```python
from build123d import *

# Parameters (mm, degrees)
SKETCH1_W                = 25.5
SKETCH1_H                = 42
BOSS_EXTRUDE1_DEPTH      = 5.5
SKETCH2_W                = 25
SKETCH2_H                = 36
CUT_EXTRUDE1_DEPTH       = 3
SKETCH3_R                = 10.5
CUT_EXTRUDE6_DEPTH       = 29
SKETCH6_R                = 2.75
CUT_EXTRUDE7_DEPTH       = 2
CUT_EXTRUDE8_DEPTH       = 13.5
CUT_EXTRUDE8_DEPTH_BACK  = 14
BOSS_EXTRUDE2_DEPTH      = 2.75
SKETCH9_R                = 2.5
CUT_EXTRUDE11_DEPTH      = 2.25
CUT_EXTRUDE12_DEPTH      = 13.5
CUT_EXTRUDE12_DEPTH_BACK = 14


with BuildPart() as part:
    # Sketch1 → Boss-Extrude1 (new body)
    with BuildSketch(Plane(origin=(0, 0, 0), x_dir=(1, 0, 0), z_dir=(0, 1, 0))):
        with Locations((-0.25, 0)):
            Rectangle(SKETCH1_W, SKETCH1_H)
    extrude(amount=BOSS_EXTRUDE1_DEPTH)

    # Sketch2 → Cut-Extrude1 (cut)
    with BuildSketch(Plane.XZ):
        with Locations((0.5, 0)):
            Rectangle(SKETCH2_W, SKETCH2_H)
    extrude(amount=-CUT_EXTRUDE1_DEPTH, mode=Mode.SUBTRACT)

    # Sketch3 → Cut-Extrude6 (cut)
    with BuildSketch(Plane(origin=(0, 13.25, -13.25), x_dir=(1, 0, 0), z_dir=(0, 0.707106781, -0.707106781))):
        with Locations((0.25, -3.789844892)):
            Circle(SKETCH3_R)
    extrude(amount=-CUT_EXTRUDE6_DEPTH, mode=Mode.SUBTRACT)

    # Sketch6 → Cut-Extrude7 (cut)
    with BuildSketch(Plane(origin=(0, 5.5, 0), x_dir=(1, 0, 0), z_dir=(0, 1, 0))):
        with Locations((-8.5, 15)):
            Circle(SKETCH6_R)
        with Locations((9, 15)):
            Circle(SKETCH6_R)
        with Locations((-8.5, -15)):
            Circle(SKETCH6_R)
        with Locations((9, -15)):
            Circle(SKETCH6_R)
    extrude(amount=-CUT_EXTRUDE7_DEPTH, mode=Mode.SUBTRACT)

    # Sketch7 → Cut-Extrude8 (cut, two sides)
    with BuildSketch(Plane(origin=(0, 0, 0), x_dir=(0, 0, -1), z_dir=(1, 0, 0))) as cut_extrude8_sk:
        Polygon((-21, 0), (-12.82380275, 9.744012446), (-21, 9.744012446), align=None)
    extrude(amount=CUT_EXTRUDE8_DEPTH, mode=Mode.SUBTRACT)
    extrude(cut_extrude8_sk.sketch, amount=-CUT_EXTRUDE8_DEPTH_BACK, mode=Mode.SUBTRACT)

    # Sketch8 → Boss-Extrude2 (add)
    with BuildSketch(Plane(origin=(-13, 0, 0), x_dir=(0, 0, -1), z_dir=(1, 0, 0))):
        Polygon((-3, 11.5), (3, 11.5), (6.464101615, 5.5), (-6.464101615, 5.5), align=None)
    extrude(amount=BOSS_EXTRUDE2_DEPTH)

    # Sketch9 → Cut-Extrude11 (cut)
    with BuildSketch(Plane(origin=(-13, 0, 0), x_dir=(0, 0, -1), z_dir=(1, 0, 0))):
        with Locations((0, 8.5)):
            Circle(SKETCH9_R)
    extrude(amount=CUT_EXTRUDE11_DEPTH, mode=Mode.SUBTRACT)

    # Sketch10 → Cut-Extrude12 (cut, two sides)
    with BuildSketch(Plane(origin=(0, 0, 0), x_dir=(0, 0, -1), z_dir=(1, 0, 0))) as cut_extrude12_sk:
        Polygon((21, 0), (15.965402213, 6), (21, 6), align=None)
    extrude(amount=CUT_EXTRUDE12_DEPTH, mode=Mode.SUBTRACT)
    extrude(cut_extrude12_sk.sketch, amount=-CUT_EXTRUDE12_DEPTH_BACK, mode=Mode.SUBTRACT)


solid = part.part
```
Source: CAD feature listing. Evaluate the final solid. Frame: model axes, mm. A direction names the side the tool comes from. Give positions to 0.01 mm unless a question says otherwise; leave off trailing zeros. Loops run counter-clockwise (first coordinate to the right, second up) from the corner with the lowest first, then second, coordinate; pieces in that order, holes last. Notation, with made-up numbers: (39.5, 61.25) - (65.5, 61.25) arc R32 ccw to (65.5, 97.25) - close; hole circle Ø11 at (12, 40). An arc over 180 degrees is marked (long way). Use CSV: the item, a comma, the result in double quotes. Start each with the question number.
1. Ray query, L1, parallel to X at y = 4.05, z = -15; L2, parallel to Y at x = -11.95, z = 0; L3, parallel to X at y = 8.5, z = -4. Return the intervals inside material, ascending.
2. Pin query (flat end, axial travel): pin 1 (2 mm diameter, centred on x = -6, y = 4, fed in from -Z); pin 2 (7.5 mm diameter, centred on x = 4, z = 1.5, fed in from +Y); pin 3 (1.5 mm diameter, centred on x = 1, y = 1.5, fed in from +Z); pin 4 (3.5 mm diameter, centred on x = 9, z = 15, fed in from +Y). Return the tip coordinate at first contact, or that it passes through.
3. Section C-C (x = 10). Output: boundary loops of the cut face in (y, z).
4. Draft query along Z for faces 4 (the cylindrical face through (-8.858, 4.514, 12.273)), 5 (the flat face through (-11.64, 8.54, -4.71)), 6 (the flat face through (-13, 3, 0)). Return one class per face: +Z half, -Z half, draft (parallel to the pull), parting line (faces both ways), or undercut.
5. Section A-A (x = -8.5). Output: boundary loops of the cut face in (y, z), then the cut area to 3 significant figures.
6. Reachability of faces 1 (the cylindrical face through (8.642, 4.514, 12.273)), 2 (the cylindrical face through (-11.89, 6.06, 0.54)), 3 (the flat face through (0, 1, -18)) from +Z, -Z, +X, -X, +Y, -Y: full face, straight path, thin tool, end or side. Return the list, or none.
7. Section B-B (y = 8.5). Output: boundary loops of the cut face in (x, z).
8. Section D-D (y = 2). Output: boundary loops of the cut face in (x, z).
Response:
1,L1,"-13 to -11.25, -5.75 to 6.25, 11.75 to 12.5"
1,L2,"3 to 6, 11 to 11.5"
1,L3,"-13 to -10.25"
2,pin 1,"z = -18.48"
2,pin 2,"through"
2,pin 3,"z = 20.37"
2,pin 4,"y = 3.5"
3,outline,"(0, -21) - (4.1, -17.56) - (3.5, -17.56) - (3.5, -12.44) - (5.5, -12.44) - (5.5, -5.65) - (3, -3.15) - (3, -18) - (0, -18) - close; (0, 18) - (3, 18) - (3, 7.87) - (5.5, 5.37) - (5.5, 12.44) - (3.5, 12.44) - (3.5, 17.56) - (4.1, 17.56) - (0, 21) - close"
4,face 4,"undercut"
4,face 5,"-Z half"
4,face 6,"draft"
5,outline,"(0, -21) - (3.87, -17.75) - (3.5, -17.75) - (3.5, -12.25) - (5.5, -12.25) - (5.5, -8.35) - (3, -5.85) - (3, -18) - (0, -18) - close; (0, 18) - (3, 18) - (3, 10.57) - (5.5, 8.07) - (5.5, 12.25) - (3.5, 12.25) - (3.5, 17.75) - (3.87, 17.75) - (0, 21) - close"
5,area,"36.8 mm²"
6,face 1,"+Y"
6,face 2,"-X"
6,face 3,"+X, -Y"
7,outline,"(-13, -4.73) - (-10.25, -4.73) - (-10.25, 4.73) - (-13, 4.73) - (-13, 2.5) - (-10.75, 2.5) - (-10.75, -2.5) - (-13, -2.5) - close"
8,outline,"(-13, -19.32) - (12.5, -19.32) - (12.5, -18) - (-12, -18) - (-12, 18) - (12.5, 18) - (12.5, 19.32) - (-13, 19.32) - close"
